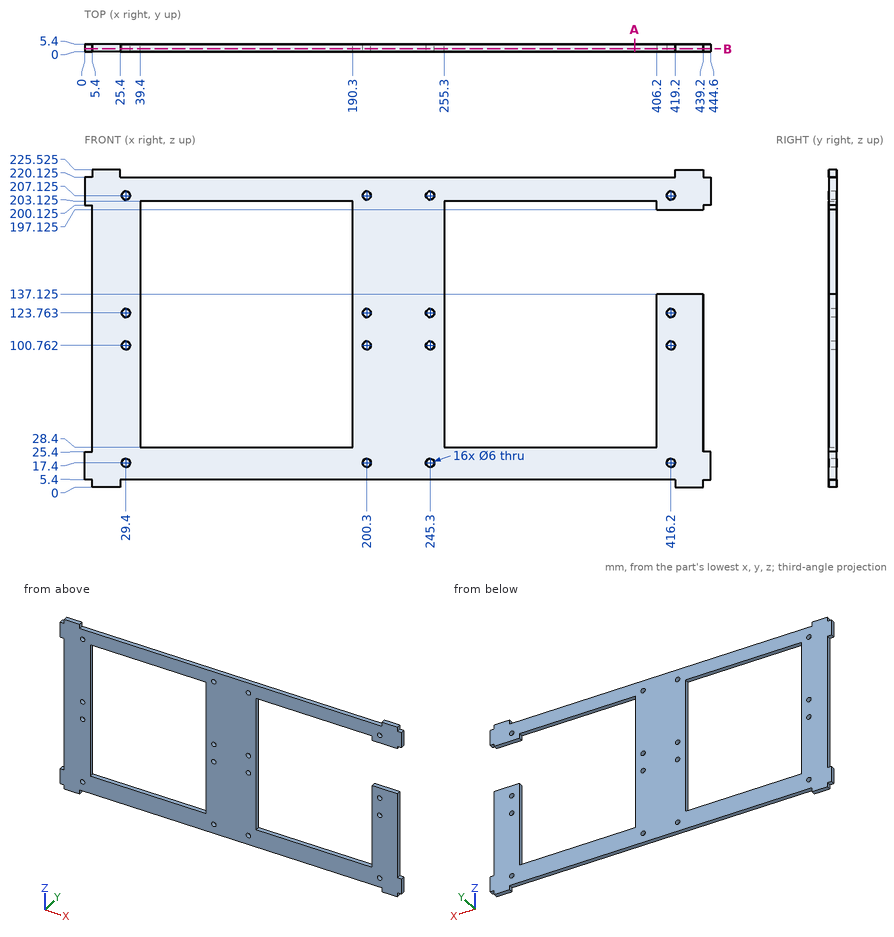
Can you work these out from the drawing? Everything is in mm from the part's minimum corner. Round coordinates to 2 decimals unless told otherwise and drop trailing zeros. Write each loop counter-clockwise with the first axis right and the second up, starting at its lowest first coordinate (ties: lowest second). Pieces come first, ordered by that corner, then holes. Notation, with made-up numbers: M -28.75,57.5 L -20.75,57.5 A25 cw -20.75,86.5 Z; hole C 38,74.25 d4. An arc over 180 degrees is marked long. Use a Markdown table: item, result.
Item 1: For pin 1 Ø1.6 at (y, z) = (4, 223) entering from +X; pin 2 Ø2.5 at (x, y) = (2, 2) entering from -Z; pin 3 Ø3 at (x, y) = (363, 1) entering from +Z (1 decimal); pin 4 Ø9.5 at (x, z) = (245.3, 100.76) entering from -Y, each with a flat end and sliding along its axis, tell me the tip position at first contact or that it passes through.
Found:
| item | result |
|---|---|
| pin 1 | stops at x = 439.2 |
| pin 2 | stops at z = 5.4 |
| pin 3 | stops at z = 220.1 |
| pin 4 | stops at y = 0 |
Item 2: I want a section at A-A (x = 390.5). List the corners of the cut face in (y, z) for me (1 decimal), and give its area (3 significant figures).
Found:
| item | result |
|---|---|
| outline | M 0,5.4 L 5.4,5.4 L 5.4,28.4 L 0,28.4 Z; M 0,203.1 L 5.4,203.1 L 5.4,220.1 L 0,220.1 Z |
| area | 216 mm2 |
Item 3: If I drill on line 1 along X through (y, z) = (5.15, 207); line 2 along Z through (x, y) = (29.4, 3.7) (1 decimal); line 3 along X through (y, z) = (1.6, 93.5), over which ranges is the centre line in solid material (lowest first)? Write a range as [from, to].
Found:
| item | result |
|---|---|
| line 1 | x = [0, 26.4], [32.4, 197.3], [203.3, 242.3], [248.3, 413.2], [419.2, 444.6] |
| line 2 | z = [5.4, 14.4], [20.4, 97.8], [103.8, 120.8], [126.8, 204.1], [210.1, 220.1] |
| line 3 | x = [5.4, 39.4], [190.3, 255.3], [406.2, 439.2] |
Item 4: I want a section at B-B (y = 1.9). State how many separate pieces and enclosed holes the cut face has.
Found:
| item | result |
|---|---|
| separate pieces | 1 |
| enclosed holes | 17 |
